Input: part model. Units: mm. Frame: model coordinates. Face numbers are marked on the shaded views. A direction names the side the tool comes from. Round coordinates to 2 decimals unless told otherwise and drop trailing zeros. Loops run counter-clockwise (first coordinate to the right, second up) from the corner with the lowest first, then second, coordinate; pieces in that order, holes last. Notation, with made-up numbers: (-16, -33.75) -> (27, -33.75) arc R27 ccw to (27, -6.75) -> close; hole circle Ø2 at (40.25, 43). An arc over 180 degrees is marked (long way). Answer as a JSON object with one key per item and string values.
```python
from build123d import *

# Parameters (mm, degrees)
SKETCH1_W                                           = 23.9
SKETCH1_H                                           = 23.9
SKETCH1_W_2                                         = 17.1
SKETCH1_H_2                                         = 17.1
BOSS_EXTRUDE1_DEPTH                                 = 15
FILLET1_R                                           = 6
SKETCH3_R                                           = 4
BOSS_EXTRUDE2_DEPTH                                 = 6
BOSS_EXTRUDE3_DEPTH                                 = 6
CBORE_FOR_M3_HEX_SOCKET_HEAD_CAP_SCREW1_D           = 3.4
CBORE_FOR_M3_HEX_SOCKET_HEAD_CAP_SCREW1_CBORE_D     = 6.5
CBORE_FOR_M3_HEX_SOCKET_HEAD_CAP_SCREW1_CBORE_DEPTH = 3.4
FILLET2_R                                           = 0.5
CSK_FOR_M3_COUNTERSUNK_FLAT_HEAD_SCREW1_D           = 3.4
CSK_FOR_M3_COUNTERSUNK_FLAT_HEAD_SCREW1_CSINK_D     = 6.3
CSK_FOR_M3_COUNTERSUNK_FLAT_HEAD_SCREW1_CSINK_ANGLE = 90


with BuildPart() as part:
    # Sketch1 → Boss-Extrude1 (new body)
    with BuildSketch(Plane.XY):
        Rectangle(SKETCH1_W, SKETCH1_H)
        Rectangle(SKETCH1_W_2, SKETCH1_H_2, mode=Mode.SUBTRACT)
    extrude(amount=BOSS_EXTRUDE1_DEPTH)

    # Fillet1
    fillet1_edges = [part.edges().sort_by_distance(p)[0] for p in [
        (11.95, -11.95, 7.5),
        (-11.95, -11.95, 7.5),
        (-11.95, 11.95, 7.5),
        (11.95, 11.95, 7.5),
    ]]
    fillet(fillet1_edges, radius=FILLET1_R)

    # Sketch3 → Boss-Extrude2 (add)
    with BuildSketch(Plane(origin=(0, 0, 0), x_dir=(-1, 0, 0), z_dir=(0, 0, -1))):
        with BuildLine():
            Line((-5.95, -11.95), (5.95, -11.95))
            ThreePointArc((5.95, -11.95), (10.192640687, -10.192640687), (11.95, -5.95))
            Line((11.95, -5.95), (11.95, 5.95))
            ThreePointArc((11.95, 5.95), (10.192640687, 10.192640687), (5.95, 11.95))
            Line((5.95, 11.95), (-5.95, 11.95))
            ThreePointArc((-5.95, 11.95), (-10.192640687, 10.192640687), (-11.95, 5.95))
            Line((-11.95, 5.95), (-11.95, -5.95))
            ThreePointArc((-11.95, -5.95), (-10.192640687, -10.192640687), (-5.95, -11.95))
        make_face()
        Circle(SKETCH3_R, mode=Mode.SUBTRACT)
    extrude(amount=-BOSS_EXTRUDE2_DEPTH)

    # Sketch2 → Boss-Extrude3 (add)
    with BuildSketch(Plane(origin=(0, 0, 0), x_dir=(-1, 0, 0), z_dir=(0, 0, -1))):
        with BuildLine():
            Line((-5.95, 11.95), (5.95, 11.95))
            ThreePointArc((5.95, 11.95), (8.773656269, 11.244049988), (10.932859145, 9.292321759))
            Line((10.932859145, 9.292321759), (4.899811493, 18.286616396))
            ThreePointArc((4.899811493, 18.286616396), (0, 20.9), (-4.899811493, 18.286616396))
            Line((-4.899811493, 18.286616396), (-10.932859145, 9.292321759))
            ThreePointArc((-10.932859145, 9.292321759), (-8.773656269, 11.244049988), (-5.95, 11.95))
        make_face()
        with BuildLine():
            Line((4.899811493, -18.286616396), (10.932859145, -9.292321759))
            ThreePointArc((10.932859145, -9.292321759), (8.773656269, -11.244049988), (5.95, -11.95))
            Line((5.95, -11.95), (-5.95, -11.95))
            ThreePointArc((-5.95, -11.95), (-8.773656269, -11.244049988), (-10.932859145, -9.292321759))
            Line((-10.932859145, -9.292321759), (-4.899811493, -18.286616396))
            ThreePointArc((-4.899811493, -18.286616396), (0, -20.9), (4.899811493, -18.286616396))
        make_face()
    extrude(amount=-BOSS_EXTRUDE3_DEPTH)

    # CBORE for M3 Hex Socket Head Cap Screw1 (through all)
    with Locations(Plane(origin=(0, 0, 0), x_dir=(-1, 0, 0), z_dir=(0, 0, -1))):
        with Locations((0, 15), (0, -15)):
            CounterBoreHole(CBORE_FOR_M3_HEX_SOCKET_HEAD_CAP_SCREW1_D / 2, CBORE_FOR_M3_HEX_SOCKET_HEAD_CAP_SCREW1_CBORE_D / 2, CBORE_FOR_M3_HEX_SOCKET_HEAD_CAP_SCREW1_CBORE_DEPTH)

    # Fillet2
    fillet2_edges = [part.edges().sort_by_distance(p)[0] for p in [
        (-11.690085142, -7.696832151, 0),
        (0, -20.9, 0),
        (7.916335319, -13.789469077, 0),
        (-7.916335319, -13.789469077, 0),
        (11.95, 0, 0),
        (-11.95, 0, 0),
        (-11.690085142, 7.696832151, 0),
        (11.690085142, -7.696832151, 0),
        (11.690085142, 7.696832151, 0),
        (-7.916335319, 13.789469077, 0),
        (0, 20.9, 0),
        (7.916335319, 13.789469077, 0),
    ]]
    fillet(fillet2_edges, radius=FILLET2_R)

    # CSK for M3 Countersunk Flat Head Screw1 (through all)
    with Locations(Plane(origin=(0, 11.95, 0), x_dir=(1, 0, 0), z_dir=(0, 1, 0))):
        with Locations((-5.2, -9.5), (5.2, -9.5)):
            CounterSinkHole(CSK_FOR_M3_COUNTERSUNK_FLAT_HEAD_SCREW1_D / 2, CSK_FOR_M3_COUNTERSUNK_FLAT_HEAD_SCREW1_CSINK_D / 2, counter_sink_angle=CSK_FOR_M3_COUNTERSUNK_FLAT_HEAD_SCREW1_CSINK_ANGLE)


solid = part.part
```
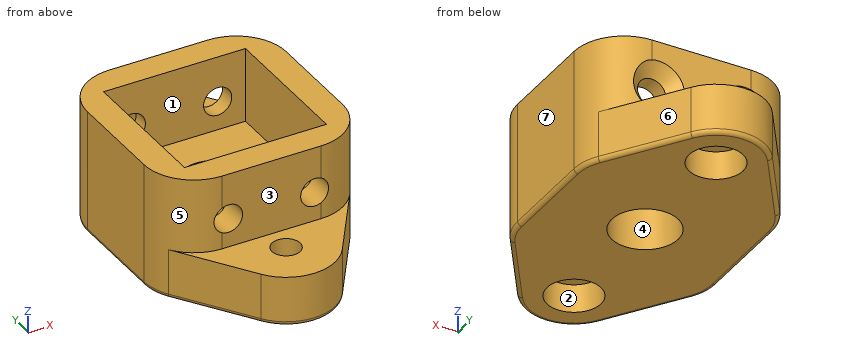
1) Contact query for flat-ended pins moving along their axis: P1, Ø5, axis at x = 3, y = 3, coming from the +Z side; P2, Ø8, axis at y = -13.5, z = 4.5, coming from the -X side; P3, Ø2.5, axis at x = -4.5, z = 11.5, coming from the -Y side. Output: stop coordinate, or through.
Output:
{"P1": "stops at z = 6", "P2": "stops at x = -10.79", "P3": "stops at y = -11.95"}
2) Reachability of the marked faces 1, 2 and 3 from +Z, -Z, +X, -X, +Y, -Y: full face, straight path, thin tool, end or side. Return the list, or none.
Output:
{"face 1": "+Z", "face 2": "-Z", "face 3": "+Z, +X, -X, -Y"}
3) Section B-B, the plane z = 2.75. Output: boundary loops of the cut face in (x, y).
Output:
{"outline": "(-11.95, -5.95) arc R6 ccw to (-10.93, -9.29) -> (-4.9, -18.29) arc R5.9 ccw to (4.9, -18.29) -> (10.93, -9.29) arc R6 ccw to (11.95, -5.95) -> (11.95, 5.95) arc R6 ccw to (10.93, 9.29) -> (4.9, 18.29) arc R5.9 ccw to (-4.9, 18.29) -> (-10.93, 9.29) arc R6 ccw to (-11.95, 5.95) -> close; hole circle Ø8 at (0, 0); hole circle Ø6.5 at (0, -15); hole circle Ø6.5 at (0, 15)"}
4) Draft query along Y for the marked faces 4, 5, 6 and 7. Return one class per face: +Y half, -Y half, draft (parallel to the pull), parting line (faces both ways), or undercut.
Output:
{"face 4": "undercut", "face 5": "-Y half", "face 6": "+Y half", "face 7": "draft"}
5) Section A-A, the plane x = 0. Count the separate pieces of the cut face and the enclosed holes in it, plus the area to 3 significant figures.
Output:
{"separate pieces": "4", "enclosed holes": "0", "area": "202 mm^2"}
6) Section C-C, the plane y = -3.5. Output: boundary loops of the cut face in (x, z), plus the area to 3 significant figures.
Output:
{"outline": "(-11.95, 0.5) arc R0.5 ccw to (-11.45, 0) -> (-1.94, 0) -> (-1.94, 6) -> (-8.55, 6) -> (-8.55, 15) -> (-11.95, 15) -> close; (1.94, 0) -> (11.45, 0) arc R0.5 ccw to (11.95, 0.5) -> (11.95, 15) -> (8.55, 15) -> (8.55, 6) -> (1.94, 6) -> close", "area": "181 mm^2"}
7) Section D-D, the plane z = 9.5. Output: boundary loops of the cut face in (x, y), plus the area to 3 significant figures.
Output:
{"outline": "(-11.95, -5.95) arc R6 ccw to (-6.9, -11.87) -> (-6.9, -8.55) -> (-8.55, -8.55) -> (-8.55, 8.55) -> (-6.9, 8.55) -> (-6.9, 10.5) -> (-7.99, 11.59) arc R6 ccw to (-11.95, 5.95) -> close; (-3.5, -11.95) -> (3.5, -11.95) -> (3.5, -8.55) -> (-3.5, -8.55) -> close; (-3.5, 8.55) -> (3.5, 8.55) -> (3.5, 10.5) -> (2.05, 11.95) -> (-2.05, 11.95) -> (-3.5, 10.5) -> close; (6.9, -11.87) arc R6 ccw to (11.95, -5.95) -> (11.95, 5.95) arc R6 ccw to (7.99, 11.59) -> (6.9, 10.5) -> (6.9, 8.55) -> (8.55, 8.55) -> (8.55, -8.55) -> (6.9, -8.55) -> close", "area": "198 mm^2"}
8) Ray query, probe 1 along X at (y, z) = (-9.85, 9.5); probe 2 along Y at (x, z) = (0, 2.45); probe 3 along Z at (x, y) = (5.2, 9.4). Return the intervals inside material, ascending.
Output:
{"probe 1": "x = -10.51 to -6.9, -3.5 to 3.5, 6.9 to 10.51", "probe 2": "y = -20.9 to -18.25, -11.75 to -4, 4 to 11.75, 18.25 to 20.9", "probe 3": "z = 0 to 7.8, 11.2 to 15"}
